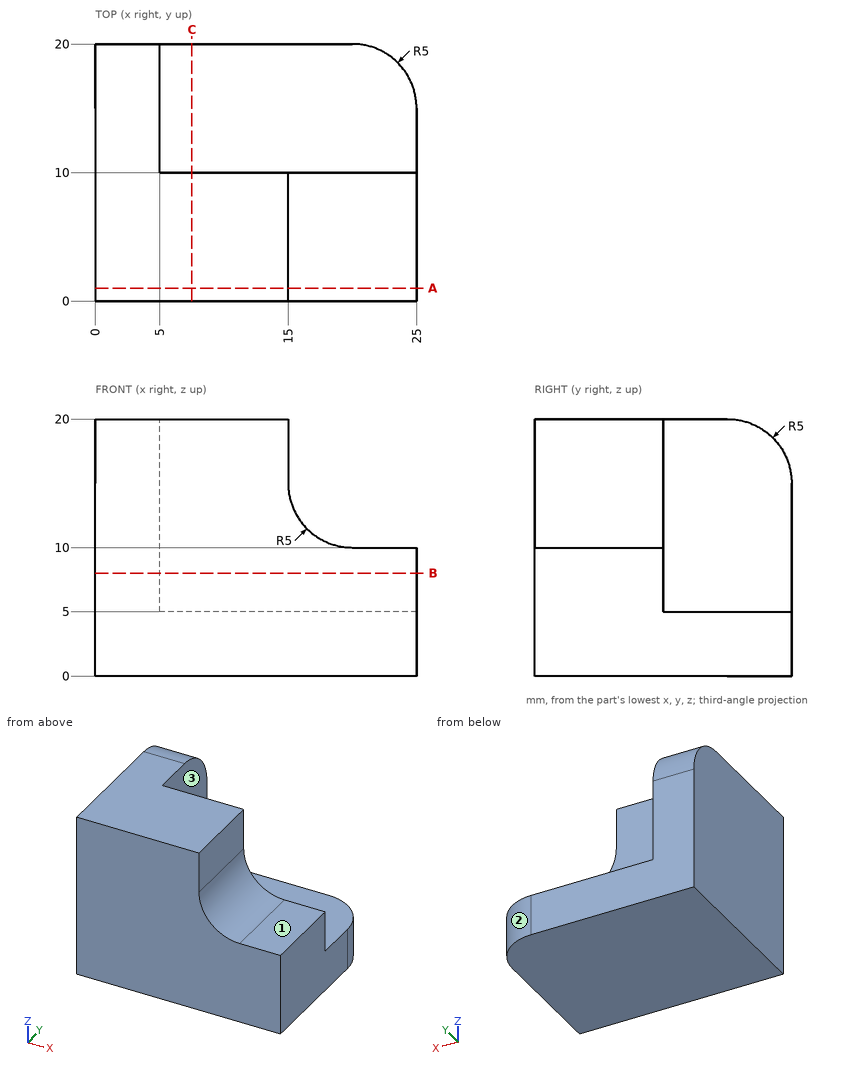
Study the drawing (mm; zero at the part's minimum x, y, z) and answer. A direction names the side the tool comes from. Give positions to 0.01 mm unless a question says otherwise; leave off trailing zeros. Loops run counter-clockwise (first coordinate to the right, second up) from the corner with the lowest first, then second, coordinate; pieces in that order, holes last. Notation, with made-up numbers: (-13, -13.75) - (15, -13.75) arc R13 ccw to (15, -5.75) - close; hole circle Ø4 at (38, -31.75). An arc over 180 degrees is marked (long way). Return JSON: item names as keys, results as strings. Group by question number.
1. Find section C-C (x = 7.5). Write down the section's boundary in (y, z).
2. Find section A-A (y = 1). Write down the section's boundary in (x, z), then the cut area to 3 significant figures.
3. Which of the six approach directions +Z, -Z, +X, -X, +Y, -Y give full straight-line access (tool end or side, diameter ignored) to the marked faces 1, 2 and 3?
4. Straight lines are drawn through the part: line 1 (Y direction, x = 16.25, z = 10); line 2 (Z direction, x = 9.75, y = 12.75). For each, find the intervals that lie inside material, in ascending order. Write a range as [from, to].
5. Given pin 1 Ø2.5 at (x, y) = (23, 4) entering from +Z; pin 2 Ø4.5 at (x, z) = (15.5, 11.5) entering from +Y; pin 3 Ø2 at (y, z) = (12, 9.5) entering from +X, each flat-ended and moving along its own axis, determine where each tip first touches the part or whether it passes through.
6. Find section B-B (z = 8). Write down the section's boundary in (x, y), then the cut area to 3 significant figures.
Verdict:
{
 "1": {"outline": "(0, 0) - (20, 0) - (20, 5) - (10, 5) - (10, 20) - (0, 20) - close"},
 "2": {"outline": "(0, 0) - (25, 0) - (25, 10) - (20, 10) arc R5 cw to (15, 15) - (15, 20) - (0, 20) - close", "area": "405 mm^2"},
 "3": {"face 1": "+Z, +X, +Y, -Y", "face 2": "+Z, -Z, +X, +Y", "face 3": "+Z, +X, +Y"},
 "4": {"line 1": "y = [0, 10]", "line 2": "z = [0, 5]"},
 "5": {"pin 1": "stops at z = 10", "pin 2": "stops at y = 10", "pin 3": "stops at x = 5"},
 "6": {"outline": "(0, 0) - (25, 0) - (25, 10) - (5, 10) - (5, 20) - (0, 20) - close", "area": "300 mm^2"}
}
